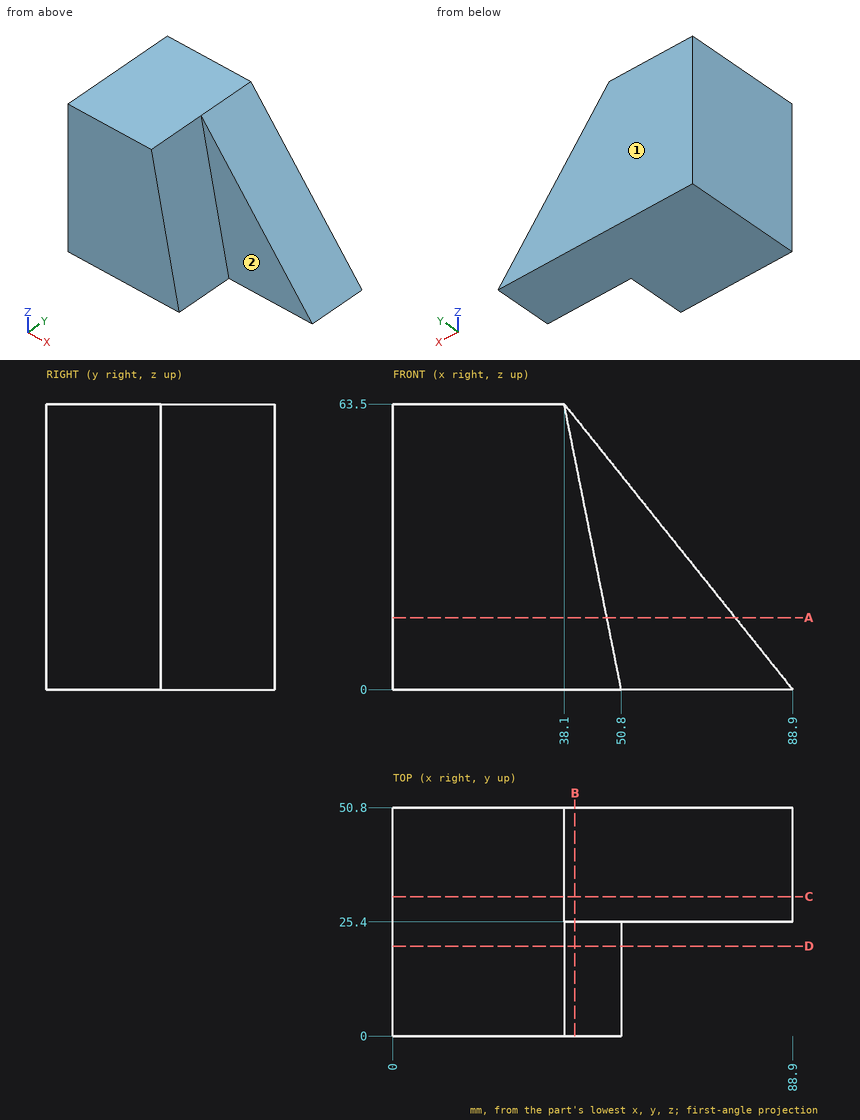
Source: three-view drawing plus pictorial views. Frame: mm from the lowest corner of the part. A direction names the side the tool comes from. Round coordinates to 2 decimals unless told otherwise and drop trailing zeros. Loops run counter-clockwise (first coordinate to the right, second up) from the corner with the lowest first, then second, coordinate; pieces in that order, holes last.
1. Access query for the marked faces 1 and 2. Directions: +Z, -Z, +X, -X, +Y, -Y. A direction counts if a zero-diameter tool reaches every point of the face in a straight line with its end or side. Return the directions, or none.
2. Section query B-B on x = 40.5. Output: boundary loops of the cut face in (y, z).
3. Contact query for flat-ended pins moving along their axis: pin 1 (8 mm diameter, centred on y = 22, z = 51.5, fed in from -X); pin 2 (8 mm diameter, centred on y = 23.5, z = 23, fed in from +X); pin 3 (10 mm diameter, centred on x = 69.5, z = 28.5, fed in from -Y). Output: stop coordinate, or through.
4. Section query D-D on y = 20. Output: boundary loops of the cut face in (x, z).
5. Section query A-A on z = 16. Output: boundary loops of the cut face in (x, y), and give its area (3 significant figures).
6. Ray query, L1, parallel to Y at x = 58.5, z = 5; L2, parallel to X at y = 14.5, z = 42.5; L3, parallel to X at y = 7, z = 28. Return the intervals inside material, ascending.
7. Section query C-C on y = 31. Output: boundary loops of the cut face in (x, z), and give its area (3 significant figures).
Answers below:
1. face 1: +Z, -Z, +X, -X, +Y
1. face 2: +Z, +X, -Y
2. outline: (0, 0) - (50.8, 0) - (50.8, 60.5) - (25.4, 60.5) - (25.4, 51.5) - (0, 51.5) - close
3. pin 1: stops at x = 0
3. pin 2: stops at x = 73.32
3. pin 3: stops at y = 25.4
4. outline: (0, 0) - (50.8, 0) - (38.1, 63.5) - (0, 63.5) - close
5. outline: (0, 0) - (47.6, 0) - (47.6, 25.4) - (76.1, 25.4) - (76.1, 50.8) - (0, 50.8) - close
5. area: 3,140 mm2
6. L1: y = 25.4 to 50.8
6. L2: x = 0 to 42.3
6. L3: x = 0 to 45.2
7. outline: (0, 0) - (88.9, 0) - (38.1, 63.5) - (0, 63.5) - close
7. area: 4,030 mm2
